Autodesk Inventor part; units mm, degrees
ref_plane "YZ Plane" through (0, 0, 0) normal (1, 0, 0) x (0, 1, 0)
ref_plane "XZ Plane" through (0, 0, 0) normal (0, 1, 0) x (-1, 0, 0)
ref_plane "XY Plane" through (0, 0, 0) normal (0, 0, 1) x (1, 0, 0)
sketch "Sketch1" plane through (0, 0, 0) normal (0, 1, 0) x (-1, 0, 0)
  line L0 (9.3536, 7.4669) -> (2.3536, 7.4669)
  line L1 (2.3536, 7.4669) -> (2.3536, 14.4669)
  line L2 (2.3536, 14.4669) -> (-4.6464, 14.4669)
  line L3 (-4.6464, 14.4669) -> (-4.6464, 21.4669)
  line L4 (-4.6464, 21.4669) -> (2.3536, 21.4669)
  line L5 (2.3536, 21.4669) -> (2.3536, 28.4669)
  line L6 (2.3536, 28.4669) -> (9.3536, 28.4669)
  line L7 (9.3536, 28.4669) -> (9.3536, 7.4669)
  point P0 (0, 0)
  dimension "d0" = 7
  dimension "d1" = 7
  dimension "d2" = 21
extrude "Plate1" add sketch "Sketch1" along normal blind 1
equation "\"d3\" = Thickness"
equation "\"BendRadius\" = Thickness"
equation "\"BendReliefWidth\" = Thickness"
equation "\"BendReliefDepth\" = 0.5 * Thickness"
equation "\"CornerReliefSize\" = 4 * Thickness"
equation "\"MinimumRemnant\" = 2 * Thickness"
equation "\"TransitionRadius\" = BendRadius"
equation "\"JacobiRadiusSize\" = BendRadius"
equation "\"GapSize\" = Thickness"
properties material "Steel, Mild"
Work out the finished part from the listing and answer in its coordinate system (mm). A direction names the side the tool comes from. Coordinates: 2 decimals unless noted, no trailing zeros. Loops run counter-clockwise (first coordinate to the right, second up) from the corner with the lowest first, then second, coordinate; pieces in that order, holes last. Notation, with made-up numbers: (14, 61) -> (66, 61) arc R6 ccw to (66, 66) -> close; hole circle Ø11 at (77.25, 48). An arc over 180 degrees is marked (long way). Answer as CSV lines item,"result".
1) For faces 1 (the face through (-9.354, 0.5, 18.1)), 2 (the face through (1.2, 0.5, 21.467)), 3 (the face through (-2.354, 0.5, 10.9)), determine the directions among +Z, -Z, +X, -X, +Y, -Y from which every point of the face is accessible in a straight line to the end or side of a thin tool.
A:
face 1,"+Z, -Z, -X, +Y, -Y"
face 2,"+Z, +X, +Y, -Y"
face 3,"-Z, +X, +Y, -Y"
2) The part is cut by section C-C (x = 2). Give the vertices of the cut face in (y, z), and give its area (3 significant figures).
A:
outline,"(0, 14.47) -> (1, 14.47) -> (1, 21.47) -> (0, 21.47) -> close"
area,"7.00 mm²"
3) The part is cut by section B-B (z = 10.25). Give the vertices of the cut face in (x, y).
A:
outline,"(-9.35, 0) -> (-2.35, 0) -> (-2.35, 1) -> (-9.35, 1) -> close"
4) Straight lines are drawn through the part: probe 1 along Z at (x, y) = (0, 0.8); probe 2 along X at (y, z) = (0.8, 9). For each, find the intervals that lie inside material, in ascending order.
A:
probe 1,"z = 14.47 to 21.47"
probe 2,"x = -9.35 to -2.35"
5) The part is cut by section A-A (y = 0.4). Give the vertices of the cut face in (x, z), and give its area (3 significant figures).
A:
outline,"(-9.35, 7.47) -> (-2.35, 7.47) -> (-2.35, 14.47) -> (4.65, 14.47) -> (4.65, 21.47) -> (-2.35, 21.47) -> (-2.35, 28.47) -> (-9.35, 28.47) -> close"
area,"196 mm²"
